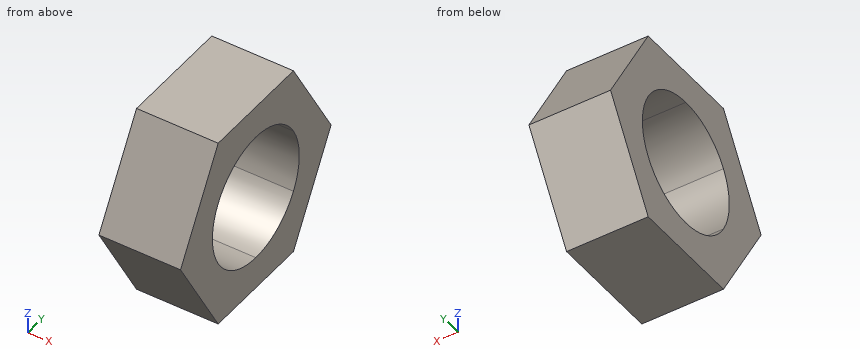
from build123d import *

# Parameters (mm, degrees)
EXTRUDE_1_DEPTH = 5


with BuildPart() as part:
    # 草图1 → 凸台-拉伸1 (new body)
    # profile 1 of 7: a face of its own
    with BuildSketch(Plane(origin=(0, 0, 0), x_dir=(0, 0, -1), z_dir=(1, 0, 0))):
        Polygon((6, -3.464101615), (6, 3.464101615), (0, 6.92820323), (-6, 3.464101615), (-6, -3.464101615), (0, -6.92820323), align=None)
        Polygon((0, -4.618802154), (4, -2.309401077), (4, 2.309401077), (0, 4.618802154), (-4, 2.309401077), (-4, -2.309401077), align=None, mode=Mode.SUBTRACT)
    # profile 2 of 7: a face of its own
    with BuildSketch(Plane(origin=(0, 0, 0), x_dir=(0, 0, -1), z_dir=(1, 0, 0))):
        with BuildLine():
            ThreePointArc((-4, 0), (-3.464101617, 1.999999997), (-2.000000006, 3.464101612))
            Line((-2.000000006, 3.464101612), (-4, 2.309401077))
            Line((-4, 2.309401077), (-4, 0))
        make_face()
    # profile 3 of 7: a face of its own
    with BuildSketch(Plane(origin=(0, 0, 0), x_dir=(0, 0, -1), z_dir=(1, 0, 0))):
        with BuildLine():
            Line((-4, -2.309401077), (-2.000000006, -3.464101612))
            ThreePointArc((-2.000000006, -3.464101612), (-3.464101617, -1.999999997), (-4, 0))
            Line((-4, 0), (-4, -2.309401077))
        make_face()
    # profile 4 of 7: a face of its own
    with BuildSketch(Plane(origin=(0, 0, 0), x_dir=(0, 0, -1), z_dir=(1, 0, 0))):
        with BuildLine():
            Line((0, -4.618802154), (2.000000006, -3.464101612))
            ThreePointArc((2.000000006, -3.464101612), (0, -4), (-2.000000006, -3.464101612))
            Line((-2.000000006, -3.464101612), (0, -4.618802154))
        make_face()
    # profile 5 of 7: a face of its own
    with BuildSketch(Plane(origin=(0, 0, 0), x_dir=(0, 0, -1), z_dir=(1, 0, 0))):
        with BuildLine():
            Line((2.000000006, -3.464101612), (4, -2.309401077))
            Line((4, -2.309401077), (4, 0))
            ThreePointArc((4, 0), (3.464101617, -1.999999997), (2.000000006, -3.464101612))
        make_face()
    # profile 6 of 7: a face of its own
    with BuildSketch(Plane(origin=(0, 0, 0), x_dir=(0, 0, -1), z_dir=(1, 0, 0))):
        with BuildLine():
            ThreePointArc((2.000000034, 3.464101596), (3.464101625, 1.999999983), (4, 0))
            Line((4, 0), (4, 2.309401077))
            Line((4, 2.309401077), (2.000000034, 3.464101596))
        make_face()
    # profile 7 of 7: a face of its own
    with BuildSketch(Plane(origin=(0, 0, 0), x_dir=(0, 0, -1), z_dir=(1, 0, 0))):
        with BuildLine():
            ThreePointArc((-2.000000006, 3.464101612), (1.6e-08, 4), (2.000000034, 3.464101596))
            Line((2.000000034, 3.464101596), (0, 4.618802154))
            Line((0, 4.618802154), (-2.000000006, 3.464101612))
        make_face()
    extrude(amount=EXTRUDE_1_DEPTH)


solid = part.part
CAD build for the part. Positions are in the model's coordinates, mm. Round coordinates to 2 decimals unless told otherwise and drop trailing zeros. Write each loop counter-clockwise with the first axis right and the second up, starting at its lowest first coordinate (ties: lowest second). Pieces come first, ordered by that corner, then holes. Notation, with made-up numbers: M -40,7.5 L 5,7.5 A30 ccw 5,45.5 Z; hole C 21,-25 d11. An arc over 180 degrees is marked long. Put each result on its own line as item: value. Start each with the question number.
1) Saw through at C-C, the plane y = -2.5. Write the cut outline in (x, z).
2) Drill centre lines: probe 1 along Z at (x, y) = (3.45, 2.75); probe 2 along Y at (x, z) = (2.7, 0.5); probe 3 along Y at (x, z) = (3.95, 3.5). Where is each one in solid material? Low to high. Write a range as [from, to].
3) Pin check, flat tips, straight feed: pin 1 Ø6 at (y, z) = (-4.5, -2) entering from -X; pin 2 Ø2 at (y, z) = (1, -2.5) entering from +X; pin 3 Ø2 at (x, z) = (2, 0.5) entering from -Y. Stop position of each tip, or through.
4) Saw through at B-B, the plane z = -3.5. Write the cut outline in (x, y), and give its area (3 significant figures).
5) Saw through at D-D, the plane z = 5.25. Write the cut outline in (x, y).
6) Saw through at A-A, the plane x = 1.4. Write the cut outline in (y, z), and give its area (3 significant figures).
Resolved:
1. outline: M 0,-6 L 5,-6 L 5,-3.12 L 0,-3.12 Z; M 0,3.12 L 5,3.12 L 5,6 L 0,6 Z
2. probe 1: [-6, -2.9], [2.9, 6]
2. probe 2: [-6.64, -3.97], [3.97, 6.64]
2. probe 3: [-4.91, -1.94], [1.94, 4.91]
3. pin 1: x = 0
3. pin 2: through
3. pin 3: y = -6.93
4. outline: M 0,-4.91 L 5,-4.91 L 5,-1.94 L 0,-1.94 Z; M 0,1.94 L 5,1.94 L 5,4.91 L 0,4.91 Z
4. area: 29.7 mm²
5. outline: M 0,-3.9 L 5,-3.9 L 5,3.9 L 0,3.9 Z
6. outline: M -6.93,0 L -3.46,-6 L 3.46,-6 L 6.93,0 L 3.46,6 L -3.46,6 Z; hole C 0,0 d8
6. area: 74.4 mm²
